from build123d import *

# Parameters (mm, degrees)
F1_DEPTH = 4.83
F2_R     = 2
F3_DEPTH = 25


with BuildPart() as f1:
    # F0 (on Top) → F1 (new body)
    with BuildSketch(Plane.XY):
        with BuildLine():
            Line((-17.055728, -14), (0, -14))
            Line((0, -14), (20.722462, -14))
            ThreePointArc((20.722462, -14), (20.952215, -13.973249), (21.169675, -13.894427))
            Line((21.169675, -13.894427), (34.447214, -7.255658))
            ThreePointArc((34.447214, -7.255658), (34.850651, -6.886962), (35, -6.361231))
            Line((35, -6.361231), (35, 10.90983))
            ThreePointArc((35, 10.90983), (34.051462, 12.611132), (32.105573, 12.698684))
            Line((32.105573, 12.698684), (18.608514, 5.950155))
            ThreePointArc((18.608514, 5.950155), (14.583592, 7.291796), (15.925233, 11.316718))
            Line((15.925233, 11.316718), (17.502942, 12.105573))
            ThreePointArc((17.502942, 12.105573), (18.028977, 13.229753), (17.055728, 14))
            Line((17.055728, 14), (0, 14))
            Line((0, 14), (-20.722462, 14))
            ThreePointArc((-20.722462, 14), (-20.952215, 13.973249), (-21.169675, 13.894427))
            Line((-21.169675, 13.894427), (-34.447214, 7.255658))
            ThreePointArc((-34.447214, 7.255658), (-34.850651, 6.886962), (-35, 6.361231))
            Line((-35, 6.361231), (-35, -10.90983))
            ThreePointArc((-35, -10.90983), (-34.051462, -12.611132), (-32.105573, -12.698684))
            Line((-32.105573, -12.698684), (-18.608514, -5.950155))
            ThreePointArc((-18.608514, -5.950155), (-14.583592, -7.291796), (-15.925233, -11.316718))
            Line((-15.925233, -11.316718), (-17.502942, -12.105573))
            ThreePointArc((-17.502942, -12.105573), (-18.028977, -13.229753), (-17.055728, -14))
        make_face()
        with BuildLine():
            ThreePointArc((0, -11), (-8.37196, -7.135145), (-10.860935, 1.743584))
            ThreePointArc((-10.860935, 1.743584), (-11.256595, 2.708251), (-12.295507, 2.796519))
            Line((-12.295507, 2.796519), (-28.552786, -5.332121))
            ThreePointArc((-28.552786, -5.332121), (-29.525731, -5.288345), (-30, -4.437694))
            Line((-30, -4.437694), (-30, 3.271061))
            ThreePointArc((-30, 3.271061), (-29.850651, 3.796792), (-29.447214, 4.165488))
            Line((-29.447214, 4.165488), (-24.92942, 6.424385))
            ThreePointArc((-24.92942, 6.424385), (-24.711959, 6.503207), (-24.482206, 6.529958))
            Line((-24.482206, 6.529958), (-9.343433, 6.529958))
            ThreePointArc((-9.343433, 6.529958), (-8.911864, 6.627878), (-8.564813, 6.902461))
            ThreePointArc((-8.564813, 6.902461), (-4.747259, 9.922879), (0, 11))
            ThreePointArc((0, 11), (8.37196, 7.135145), (10.860935, -1.743584))
            ThreePointArc((10.860935, -1.743584), (11.256595, -2.708251), (12.295507, -2.796519))
            Line((12.295507, -2.796519), (28.552786, 5.332121))
            ThreePointArc((28.552786, 5.332121), (29.525731, 5.288345), (30, 4.437694))
            Line((30, 4.437694), (30, -3.271061))
            ThreePointArc((30, -3.271061), (29.850651, -3.796792), (29.447214, -4.165488))
            Line((29.447214, -4.165488), (24.92942, -6.424385))
            ThreePointArc((24.92942, -6.424385), (24.711959, -6.503207), (24.482206, -6.529958))
            Line((24.482206, -6.529958), (9.343433, -6.529958))
            ThreePointArc((9.343433, -6.529958), (8.911864, -6.627878), (8.564813, -6.902461))
            ThreePointArc((8.564813, -6.902461), (4.747259, -9.922879), (0, -11))
        make_face(mode=Mode.SUBTRACT)
    extrude(amount=F1_DEPTH)

    # F2 (on face) → F3 (cut)
    with BuildSketch(Plane.XY.offset(4.83)):
        with Locations((-18, 15)):
            Circle(F2_R)
        with BuildLine():
            ThreePointArc((16, 15), (14, 17), (12, 15))
            ThreePointArc((12, 15), (14, 13), (16, 15))
        make_face()
        with BuildLine():
            ThreePointArc((12, 15), (10, 17), (8, 15))
            ThreePointArc((8, 15), (10, 13), (12, 15))
        make_face()
        with BuildLine():
            ThreePointArc((8, 15), (6, 17), (4, 15))
            ThreePointArc((4, 15), (6, 13), (8, 15))
        make_face()
        with BuildLine():
            ThreePointArc((4, 15), (2, 17), (0, 15))
            ThreePointArc((0, 15), (2, 13), (4, 15))
        make_face()
        with BuildLine():
            ThreePointArc((0, 15), (-2, 17), (-4, 15))
            ThreePointArc((-4, 15), (-2, 13), (0, 15))
        make_face()
        with BuildLine():
            ThreePointArc((-4, 15), (-6, 17), (-8, 15))
            ThreePointArc((-8, 15), (-6, 13), (-4, 15))
        make_face()
        with BuildLine():
            ThreePointArc((-8, 15), (-10, 17), (-12, 15))
            ThreePointArc((-12, 15), (-10, 13), (-8, 15))
        make_face()
        with BuildLine():
            ThreePointArc((-12, 15), (-14, 17), (-16, 15))
            ThreePointArc((-16, 15), (-14, 13), (-12, 15))
        make_face()
        with BuildLine():
            ThreePointArc((0, -15), (2, -17), (4, -15))
            ThreePointArc((4, -15), (2, -13), (0, -15))
        make_face()
        with Locations((-14, -15)):
            Circle(F2_R)
        with BuildLine():
            ThreePointArc((-12, -15), (-10, -17), (-8, -15))
            ThreePointArc((-8, -15), (-10, -13), (-12, -15))
        make_face()
        with BuildLine():
            ThreePointArc((-8, -15), (-6, -17), (-4, -15))
            ThreePointArc((-4, -15), (-6, -13), (-8, -15))
        make_face()
        with BuildLine():
            ThreePointArc((-4, -15), (-2, -17), (0, -15))
            ThreePointArc((0, -15), (-2, -13), (-4, -15))
        make_face()
        with BuildLine():
            ThreePointArc((20, -15), (18, -13), (16, -15))
            ThreePointArc((16, -15), (18, -17), (20, -15))
        make_face()
        with BuildLine():
            ThreePointArc((16, -15), (14, -13), (12, -15))
            ThreePointArc((12, -15), (14, -17), (16, -15))
        make_face()
        with BuildLine():
            ThreePointArc((12, -15), (10, -13), (8, -15))
            ThreePointArc((8, -15), (10, -17), (12, -15))
        make_face()
        with BuildLine():
            ThreePointArc((8, -15), (6, -13), (4, -15))
            ThreePointArc((4, -15), (6, -17), (8, -15))
        make_face()
    extrude(amount=-F3_DEPTH, mode=Mode.SUBTRACT)


solid = f1.part
Input: part model. Units: mm. Frame: model coordinates. A direction names the side the tool comes from. Round coordinates to 2 decimals unless told otherwise and drop trailing zeros. Order: outer loops, then holes, each group sorted by start corner. A loop starts at its lowest first (then second) coordinate and runs counter-clockwise, first axis right, second up. Notation, with made-up numbers: (-16.75, 67.5) - (-10.75, 67.5) arc R21 cw to (-10.75, 84.5) - close; hole circle Ø6 at (20.5, -4). An arc over 180 degrees is marked (long way). Use a Markdown table: item, result.
1. Access query for faces 4 (the face through (25.45, 9.37, 2.38)), 5 (the face through (-18.033, -13.211, 2.381)), 6 (the face through (14, -13, 2)). Directions: +Z, -Z, +X, -X, +Y, -Y. A direction counts if a zero-diameter tool reaches every point of the face in a straight line with its end or side. Return the directions, or none.
Evaluation:
| item | result |
|---|---|
| face 4 | +Z, -Z, +Y |
| face 5 | +Z, -Z |
| face 6 | +Z, -Z, -Y |
2. Section B-B on x = -6. Return the cut outline in (y, z).
Evaluation:
| item | result |
|---|---|
| outline | (-13, 0) - (-9.22, 0) - (-9.22, 4.83) - (-13, 4.83) - close; (9.22, 0) - (13, 0) - (13, 4.83) - (9.22, 4.83) - close |
3. Material intervals for probe 1 along X at (y, z) = (4, 1.35); probe 2 along X at (y, z) = (2, 2.55); probe 3 along Y at (x, z) = (-15.5, 4.6), sorted ascending.
Evaluation:
| item | result |
|---|---|
| probe 1 | -35 to -29.68, 10.25 to 25.89, 30 to 35 |
| probe 2 | -35 to -30, -13.89 to -10.85, 10.82 to 21.89, 30 to 35 |
| probe 3 | -13.68 to -11.06, -6.21 to 1.19, 6.53 to 13.68 |
4. Section A-A on y = 10. Return the cut outline in (x, z), then the cut area to 3 significant figures.
Evaluation:
| item | result |
|---|---|
| outline | (-28.96, 0) - (-4.58, 0) - (-4.58, 4.83) - (-28.96, 4.83) - close; (4.58, 0) - (14.6, 0) - (14.6, 4.83) - (4.58, 4.83) - close; (26.71, 0) - (35, 0) - (35, 4.83) - (26.71, 4.83) - close |
| area | 206 mm^2 |
5. Mould query, pull axis Y, two halves, no side actions, for faces 1 (the face through (-10, 13, 2)), 2 (the face through (17, -6.53, 2)), 3 (the face through (-10, -13, 2)). Classes: +Y half, -Y half, draft (parallel to the pull), parting line (faces both ways), or undercut.
Evaluation:
| item | result |
|---|---|
| face 1 | +Y half |
| face 2 | undercut |
| face 3 | -Y half |
6. Section C-C on y = 0.5. Return the cut outline in (x, z), then the cut area to 3 significant figures.
Evaluation:
| item | result |
|---|---|
| outline | (-35, 0) - (-30, 0) - (-30, 4.83) - (-35, 4.83) - close; (-16.89, 0) - (-10.99, 0) - (-10.99, 4.83) - (-16.89, 4.83) - close; (10.99, 0) - (18.89, 0) - (18.89, 4.83) - (10.99, 4.83) - close; (30, 0) - (35, 0) - (35, 4.83) - (30, 4.83) - close |
| area | 115 mm^2 |
7. First-contact query: pin 1 (1.5 mm diameter, centred on x = -19, z = 1, fed in from -Y); pin 2 (1 mm diameter, centred on x = 14.5, z = 1, fed in from -Y). Flat tips, straight axial feed; report the tip coordinate or a pass-through.
Evaluation:
| item | result |
|---|---|
| pin 1 | y = -6.52 |
| pin 2 | y = -13.27 |
8. Section D-D on x = 22. Return the cut outline in (y, z), then the cut area to 3 significant figures.
Evaluation:
| item | result |
|---|---|
| outline | (-13.48, 0) - (-6.53, 0) - (-6.53, 4.83) - (-13.48, 4.83) - close; (2.06, 0) - (7.65, 0) - (7.65, 4.83) - (2.06, 4.83) - close |
| area | 60.6 mm^2 |
